Geometry: final body of the model. Coordinates: model frame, mm. A direction names the side the tool comes from. Give positions to 0.01 mm unless a question says otherwise; leave off trailing zeros. Write each loop counter-clockwise with the first axis right and the second up, starting at its lowest first coordinate (ties: lowest second). Pieces come first, ordered by that corner, then holes.
from build123d import *

# Parameters (mm, degrees)
F0_W          = 900
F0_H          = 500
F1_DEPTH      = 28
F2_R          = 10
F3_DEPTH      = 25
F3_DEPTH_BACK = 35
F4_DEPTH      = 25
F4_DEPTH_BACK = 35
F6_W          = 17
F6_H          = 500
F7_DEPTH      = 11
F9_DEPTH      = 25
F9_DEPTH_BACK = 35
F10_R         = 8
F11_W         = 866
F11_H         = 17
F12_DEPTH     = 11
F13_W         = 300
F13_H         = 27
F14_DEPTH     = 8


with BuildPart() as f1:
    # F0 (on Front) → F1 (new body)
    with BuildSketch(Plane.XZ):
        Rectangle(F0_W, F0_H)
    extrude(amount=F1_DEPTH)


with BuildPart() as f3:
    # F2 (on face) → F3 (new body, two sides)
    with BuildSketch(Plane.XZ.offset(28)) as f3_sk:
        with Locations((300, -100)):
            Circle(F2_R)
        with Locations((200, -100)):
            Circle(F2_R)
        with Locations((100, -100)):
            Circle(F2_R)
        with Locations((0, -100)):
            Circle(F2_R)
        with Locations((-100, -100)):
            Circle(F2_R)
        with Locations((-200, -100)):
            Circle(F2_R)
        with Locations((-300, -100)):
            Circle(F2_R)
        with Locations((-400, -100)):
            Circle(F2_R)
        with Locations((-400, 0)):
            Circle(F2_R)
        with Locations((-300, 0)):
            Circle(F2_R)
        with Locations((-200, 0)):
            Circle(F2_R)
        with Locations((-100, 0)):
            Circle(F2_R)
        Circle(F2_R)
        with Locations((100, 0)):
            Circle(F2_R)
        with Locations((200, 0)):
            Circle(F2_R)
        with Locations((300, 0)):
            Circle(F2_R)
        with Locations((-400, 100)):
            Circle(F2_R)
        with Locations((-300, 100)):
            Circle(F2_R)
        with Locations((-200, 100)):
            Circle(F2_R)
        with Locations((-100, 100)):
            Circle(F2_R)
        with Locations((0, 100)):
            Circle(F2_R)
        with Locations((100, 100)):
            Circle(F2_R)
        with Locations((200, 100)):
            Circle(F2_R)
        with Locations((300, 100)):
            Circle(F2_R)
        with Locations((-400, 200)):
            Circle(F2_R)
        with Locations((-300, 200)):
            Circle(F2_R)
        with Locations((-200, 200)):
            Circle(F2_R)
        with Locations((-100, 200)):
            Circle(F2_R)
        with Locations((0, 200)):
            Circle(F2_R)
        with Locations((100, 200)):
            Circle(F2_R)
        with Locations((200, 200)):
            Circle(F2_R)
        with Locations((300, 200)):
            Circle(F2_R)
    extrude(amount=F3_DEPTH)
    extrude(f3_sk.sketch, amount=-F3_DEPTH_BACK)


with BuildPart() as f4:
    # F2 (on face) → F4 (new body, two sides)
    with BuildSketch(Plane.XZ.offset(28)) as f4_sk:
        with Locations((300, -100)):
            Circle(F2_R)
        with Locations((200, -100)):
            Circle(F2_R)
        with Locations((100, -100)):
            Circle(F2_R)
        with Locations((0, -100)):
            Circle(F2_R)
        with Locations((-100, -100)):
            Circle(F2_R)
        with Locations((-200, -100)):
            Circle(F2_R)
        with Locations((-300, -100)):
            Circle(F2_R)
        with Locations((-400, -100)):
            Circle(F2_R)
        with Locations((-400, 0)):
            Circle(F2_R)
        with Locations((-300, 0)):
            Circle(F2_R)
        with Locations((-200, 0)):
            Circle(F2_R)
        with Locations((-100, 0)):
            Circle(F2_R)
        Circle(F2_R)
        with Locations((100, 0)):
            Circle(F2_R)
        with Locations((200, 0)):
            Circle(F2_R)
        with Locations((300, 0)):
            Circle(F2_R)
        with Locations((-400, 100)):
            Circle(F2_R)
        with Locations((-300, 100)):
            Circle(F2_R)
        with Locations((-200, 100)):
            Circle(F2_R)
        with Locations((-100, 100)):
            Circle(F2_R)
        with Locations((0, 100)):
            Circle(F2_R)
        with Locations((100, 100)):
            Circle(F2_R)
        with Locations((200, 100)):
            Circle(F2_R)
        with Locations((300, 100)):
            Circle(F2_R)
        with Locations((-400, 200)):
            Circle(F2_R)
        with Locations((-300, 200)):
            Circle(F2_R)
        with Locations((-200, 200)):
            Circle(F2_R)
        with Locations((-100, 200)):
            Circle(F2_R)
        with Locations((0, 200)):
            Circle(F2_R)
        with Locations((100, 200)):
            Circle(F2_R)
        with Locations((200, 200)):
            Circle(F2_R)
        with Locations((300, 200)):
            Circle(F2_R)
    extrude(amount=F4_DEPTH)
    extrude(f4_sk.sketch, amount=-F4_DEPTH_BACK)


with BuildPart() as f1_1:
    add(f1.part)

    # F5: cut F3, F4
    add(f3.part, mode=Mode.SUBTRACT)
    add(f4.part, mode=Mode.SUBTRACT)

    # F6 (on face) → F7 (cut)
    with BuildSketch(Plane.XZ.offset(28)):
        with Locations((441.5, 0)):
            Rectangle(F6_W, F6_H)
        with Locations((-441.5, 0)):
            Rectangle(F6_W, F6_H)
    extrude(amount=-F7_DEPTH, mode=Mode.SUBTRACT)

    # F8 (on face) → F9 (cut, two sides)
    with BuildSketch(Plane.XZ.offset(28)) as f9_sk:
        with BuildLine():
            Line((415, -197.5), (415, -117.5))
            ThreePointArc((415, -117.5), (397.5, -100), (380, -117.5))
            Line((380, -117.5), (380, -197.5))
            ThreePointArc((380, -197.5), (397.5, -215), (415, -197.5))
        make_face()
        with BuildLine():
            Line((414.999995, 117.5), (414.999995, 197.5))
            ThreePointArc((414.999995, 197.5), (397.499995, 215), (379.999995, 197.5))
            Line((379.999995, 197.5), (379.999995, 117.5))
            ThreePointArc((379.999995, 117.5), (397.499995, 100), (414.999995, 117.5))
        make_face()
    extrude(amount=F9_DEPTH, mode=Mode.SUBTRACT)
    extrude(f9_sk.sketch, amount=-F9_DEPTH_BACK, mode=Mode.SUBTRACT)

    # F10
    f10_edges = [f1_1.edges().sort_by_distance(p)[0] for p in [
        (397.499995, -28, 100),
        (397.499995, 0, 100),
        (397.5, -28, -215),
        (397.5, 0, -215),
    ]]
    fillet(f10_edges, radius=F10_R)

    # F11 (on face) → F12 (cut)
    with BuildSketch(Plane.XZ.offset(28)):
        with Locations((0, -241.5)):
            Rectangle(F11_W, F11_H)
    extrude(amount=-F12_DEPTH, mode=Mode.SUBTRACT)

    # F13 (on face) → F14 (cut)
    with BuildSketch(Plane.XZ.offset(17)):
        with Locations((0, -236.5)):
            Rectangle(F13_W, F13_H)
    extrude(amount=-F14_DEPTH, mode=Mode.SUBTRACT)


solid = f1_1.part
Q1. Access query for faces 1 (the flat face through (-2, -9, -236)), 2 (the cylindrical face through (397.115, -14.084, -214.996)). Directions: +Z, -Z, +X, -X, +Y, -Y. A direction counts if a zero-diameter tool reaches every point of the face in a straight line with its end or side. Return the directions, or none.
Filled sheet:
face 1: -Z
face 2: +Y, -Y
Q2. Pull-direction query (X, two-part tool) for faces 3 (the flat face through (-450, -8, -3)), 4 (the flat face through (-6, -8, -250)), 5 (the cylindrical face through (397.115, -14.084, 100.004)); classes: released by +X, released by -X, zero draft, split by the parting line, or undercut.
Filled sheet:
face 3: released by -X
face 4: zero draft
face 5: undercut
Q3. Section A-A on x = -400. Output: boundary loops of the cut face in (y, z).
Filled sheet:
outline: (-28, -233) - (-17, -233) - (-17, -250) - (0, -250) - (0, -110) - (-28, -110) - close; (-28, -90) - (0, -90) - (0, -10) - (-28, -10) - close; (-28, 10) - (0, 10) - (0, 90) - (-28, 90) - close; (-28, 110) - (0, 110) - (0, 190) - (-28, 190) - close; (-28, 210) - (0, 210) - (0, 250) - (-28, 250) - close
Q4. Pin query (flat end, axial travel): P1, Ø8, axis at x = 24.5, y = -14, coming from the -Z side; P2, Ø16, axis at x = 100, z = 0, coming from the +Y side; P3, Ø2, axis at x = 125.5, y = -14.5, coming from the -Z side. Return the tip coordinate at first contact, or that it passes through.
Filled sheet:
P1: stops at z = -233
P2: passes through
P3: stops at z = -223
Q5. Section B-B on x = 397.5. Count the separate pieces of the cut face and the enclosed holes in it, plus the area to 3 significant figures.
Filled sheet:
separate pieces: 3
enclosed holes: 0
area: 7,260 mm2
Q6. Ray query, line 1 along Z through (x, y) = (-400, -8.25); line 2 along Z through (x, y) = (100, -22.5); line 3 along X through (y, z) = (-19.75, 137). Return the intervals inside material, ascending.
Filled sheet:
line 1: z = -250 to -110, -90 to -10, 10 to 90, 110 to 190, 210 to 250
line 2: z = -233 to -110, -90 to -10, 10 to 90, 110 to 190, 210 to 250
line 3: x = -433 to 380, 415 to 433
